```python
from build123d import *

# Parameters (mm, degrees)
SKETCH1_W                   = 80
SKETCH1_H                   = 12.7
BOSS_EXTRUDE1_DEPTH         = 12.7
CUT_EXTRUDE1_DEPTH          = 44.847234804
M4_TAPPED_HOLE2_D           = 3.3
M4_TAPPED_HOLE2_CSINK_D     = 4.05
M4_TAPPED_HOLE2_CSINK_ANGLE = 90
M5_TAPPED_HOLE1_D           = 4.2
M5_TAPPED_HOLE1_CSINK_D     = 5.05
M5_TAPPED_HOLE1_CSINK_ANGLE = 90


with BuildPart() as part:
    # Sketch1 → Boss-Extrude1 (new body)
    with BuildSketch(Plane(origin=(0, 0, 0), x_dir=(1, 0, 0), z_dir=(0, 1, 0))):
        Rectangle(SKETCH1_W, SKETCH1_H)
    extrude(amount=BOSS_EXTRUDE1_DEPTH)

    # Sketch4 → Cut-Extrude1 (cut, through all)
    with BuildSketch(Plane.XY.offset(6.35)):
        with BuildLine():
            ThreePointArc((0, 2.593672006), (8.3, 6.35), (0, 10.106327994))
            ThreePointArc((0, 10.106327994), (-8.3, 6.35), (0, 2.593672006))
        make_face()
    extrude(amount=-CUT_EXTRUDE1_DEPTH, mode=Mode.SUBTRACT)

    # M4 Tapped Hole2 (through all)
    with Locations(Plane(origin=(0, 12.7, 0), x_dir=(1, 0, 0), z_dir=(0, 1, 0))):
        with Locations((-35, 0), (-20, 0)):
            CounterSinkHole(M4_TAPPED_HOLE2_D / 2, M4_TAPPED_HOLE2_CSINK_D / 2, counter_sink_angle=M4_TAPPED_HOLE2_CSINK_ANGLE)

    # M5 Tapped Hole1 (through all)
    with Locations(Plane(origin=(0, 12.7, 0), x_dir=(1, 0, 0), z_dir=(0, 1, 0))):
        with Locations((35, 0), (20, 0)):
            CounterSinkHole(M5_TAPPED_HOLE1_D / 2, M5_TAPPED_HOLE1_CSINK_D / 2, counter_sink_angle=M5_TAPPED_HOLE1_CSINK_ANGLE)


solid = part.part
```
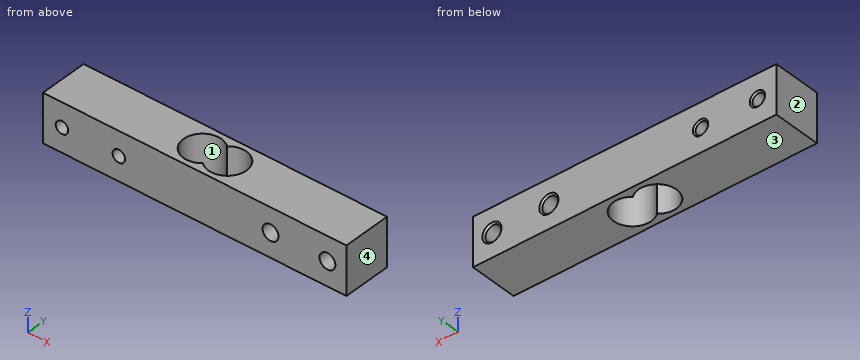
CAD build for the part. Positions are in the model's coordinates, mm. Face numbers are marked on the shaded views. Coordinates: 2 decimals unless noted, no trailing zeros. Loops run counter-clockwise (first coordinate to the right, second up) from the corner with the lowest first, then second, coordinate; pieces in that order, holes last. Notation, with made-up numbers: (35.25, 62) - (86.25, 62) arc R25 ccw to (86.25, 100) - close; hole circle Ø6 at (37.5, 37.25). An arc over 180 degrees is marked (long way). Use CSV: the item, a comma, the result in double quotes. Start each with the question number.
Q1. Cut at D-D, the plane x = -3.3. List the corners of the cut face in (y, z), then the cut area to 3 significant figures.
Q2. Probe probe 1 along X at (y, z) = (6, 4.75); probe 2 along Y at (x, z) = (-3.3, -1); probe 3 along Z at (x, y) = (20, 8). List the from-to ranges inside material, lowest first. Write a range as from..to.
Q3. Cut at C-C, the plane z = 0. State how many separate pieces and enclosed holes the cut face has, then the cut area to 3 significant figures.
Q4. Cut at B-B, the plane y = 6.5. List the corners of the cut face in (x, z), then the cut area to 3 significant figures.
Q5. Two-plate mould, pull along X, no slides. Class the marked faces 1, 2, 3 and 4: +X half, -X half, draft (parallel to the pull), parting line (faces both ways), or undercut.
Q6. Cut at A-A, the plane x = 35. List the corners of the cut face in (y, z) (3 decimals).
Here are the results:
1,outline,"(0, -6.35) - (1.35, -6.35) - (1.35, 6.35) - (0, 6.35) - close; (11.35, -6.35) - (12.7, -6.35) - (12.7, 6.35) - (11.35, 6.35) - close"
1,area,"34.3 mm2"
2,probe 1,"-40..-8.29, 8.29..40"
2,probe 2,"0..1.35, 11.35..12.7"
2,probe 3,"-6.35..-2.1, 2.1..6.35"
3,separate pieces,"5"
3,enclosed holes,"1"
3,area,"685 mm2"
4,outline,"(-40, -6.35) - (-8.3, -6.35) - (-8.3, 6.35) - (-40, 6.35) - close; (8.3, -6.35) - (40, -6.35) - (40, 6.35) - (8.3, 6.35) - close; hole circle Ø3.3 at (-35, 0); hole circle Ø3.3 at (-20, 0); hole circle Ø4.2 at (20, 0); hole circle Ø4.2 at (35, 0)"
4,area,"760 mm2"
5,face 1,"undercut"
5,face 2,"-X half"
5,face 3,"draft"
5,face 4,"+X half"
6,outline,"(0, -6.35) - (12.7, -6.35) - (12.7, -2.525) - (12.275, -2.1) - (0, -2.1) - close; (0, 2.1) - (12.275, 2.1) - (12.7, 2.525) - (12.7, 6.35) - (0, 6.35) - close"
